Geometry: final body of the model. Coordinates: model frame, mm. A direction names the side the tool comes from. Give positions to 0.01 mm unless a question says otherwise; leave off trailing zeros. Write each loop counter-clockwise with the first axis right and the second up, starting at its lowest first coordinate (ties: lowest second). Pieces come first, ordered by that corner, then holes.
Q1. Reachability of faces 4 (the flat face through (15, -51, 0)), 5 (the flat face through (-1, 6, 4)), 6 (the flat face through (11, -54, 8)) from +Z, -Z, +X, -X, +Y, -Y: full face, straight path, thin tool, end or side. Return the list, or none.
Q2. Section C-C (y = -15.5). Return the cut outline in (x, z), plus the area to 3 significant figures.
Q3. Pin query (flat end, axial travel): pin 1 Ø2 at (x, z) = (8, 10.5) entering from +Y; pin 2 Ø3 at (y, z) = (1, 7) entering from -X; pin 3 Ø2 at (y, z) = (-28.5, -13) entering from -X. Return the tip coordinate at first contact, or that it passes through.
Q4. Section A-A (z = 0). Return the cut outline in (x, y), plus the area to 3 significant figures.
Q5. Section B-B (x = 0). Return the cut outline in (y, z), plus the area to 3 significant figures.
Q6. Line query: line 1 (Y direction, x = -12, z = 2.5); line 2 (Y direction, x = -13.5, z = -11.5); line 3 (Z direction, x = 13.5, y = -55). Output: solid intervals per line, ascending.
Q7. Section D-D (x = -7). Return the cut outline in (y, z), plus the area to 3 significant figures.
Q8. Mould query, pull axis X, two halves, no side actions, for faces 1 (the cylindrical face through (1.352, -55.19, 4.292)), 2 (the flat face through (11, -56.5, 0)), 3 (the cylindrical face through (-16.108, -38.325, -3.577)). Classes: +X half, -X half, draft (parallel to the pull), parting line (faces both ways), or undercut.
from build123d import *

# Parameters (mm, degrees)
SKETCH1_R           = 18.5
SKETCH1_R_2         = 16.5
SKETCH1_R_3         = 6
SKETCH1_R_4         = 4.5
SKETCH1_W           = 6
SKETCH1_H           = 16
SKETCH1_R_5         = 3
BOSS_EXTRUDE1_DEPTH = 26
BOSS_EXTRUDE2_START = -26
SKETCH1_3_R         = 16.5
BOSS_EXTRUDE2_DEPTH = 25
BOSS_EXTRUDE3_START = -56.5
SKETCH1_4_W         = 6
SKETCH1_4_H         = 16
BOSS_EXTRUDE3_DEPTH = 5.5
BOSS_EXTRUDE4_START = -51
SKETCH1_5_R         = 4.5
BOSS_EXTRUDE4_DEPTH = 8.5
SKETCH1_6_R         = 6
BOSS_EXTRUDE5_DEPTH = 6
BOSS_EXTRUDE6_START = 6
SKETCH1_7_R         = 3
BOSS_EXTRUDE6_DEPTH = 15


with BuildPart() as part:
    # Sketch1 → Boss-Extrude1 (new body)
    # profile 1 of 14: a face of its own
    with BuildSketch(Plane(origin=(0, 0, 0), x_dir=(1, 0, 0), z_dir=(0, 1, 0))):
        with Locations(Location((0, 0, 0), (0, 0, 270))):
            Circle(SKETCH1_R)
        Circle(SKETCH1_R_2, mode=Mode.SUBTRACT)
    # profile 2 of 14: a face of its own
    with BuildSketch(Plane(origin=(0, 0, 0), x_dir=(1, 0, 0), z_dir=(0, 1, 0))):
        with BuildLine():
            Line((14.43086969, -8), (8.43086969, -8))
            Line((8.43086969, -8), (8.43086969, 8))
            Line((8.43086969, 8), (14.43086969, 8))
            ThreePointArc((14.43086969, 8), (-16.5, 0), (14.43086969, -8))
        make_face()
        with BuildLine():
            ThreePointArc((3.822221213, -2.375), (5.428320517, -4.443960806), (6, -7))
            ThreePointArc((6, -7), (-2.556039194, -12.428320517), (-3.822221213, -2.375))
            ThreePointArc((-3.822221213, -2.375), (-1.234909823, 4.327239042), (4.5, 0))
            ThreePointArc((4.5, 0), (4.327239042, -1.234909823), (3.822221213, -2.375))
        make_face(mode=Mode.SUBTRACT)
    # profile 3 of 14: a face of its own
    with BuildSketch(Plane(origin=(0, 0, 0), x_dir=(1, 0, 0), z_dir=(0, 1, 0))):
        with Locations((0, -7)):
            Circle(SKETCH1_R_3)
    # profile 4 of 14: a face of its own
    with BuildSketch(Plane(origin=(0, 0, 0), x_dir=(1, 0, 0), z_dir=(0, 1, 0))):
        Circle(SKETCH1_R_4)
    # profile 5 of 14: a face of its own
    with BuildSketch(Plane(origin=(0, 0, 0), x_dir=(1, 0, 0), z_dir=(0, 1, 0))):
        with Locations((11.43086969, 0)):
            Rectangle(SKETCH1_W, SKETCH1_H)
    # profile 6 of 14: a face of its own
    with BuildSketch(Plane(origin=(0, 0, 0), x_dir=(1, 0, 0), z_dir=(0, 1, 0))):
        with BuildLine():
            Line((14.43086969, 8), (14.43086969, -8))
            ThreePointArc((14.43086969, -8), (15.974344273, -4.13162499), (16.5, 0))
            ThreePointArc((16.5, 0), (15.974344273, 4.13162499), (14.43086969, 8))
        make_face()
    # profile 7 of 14: a face of its own
    with BuildSketch(Plane(origin=(0, 0, 0), x_dir=(1, 0, 0), z_dir=(0, 1, 0))):
        Circle(SKETCH1_R_4)
    # profile 8 of 14: a face of its own
    with BuildSketch(Plane(origin=(0, 0, 0), x_dir=(1, 0, 0), z_dir=(0, 1, 0))):
        with Locations((0, -7)):
            Circle(SKETCH1_R_3)
        with Locations((0, -7)):
            Circle(SKETCH1_R_5, mode=Mode.SUBTRACT)
    # profile 9 of 14: a face of its own
    with BuildSketch(Plane(origin=(0, 0, 0), x_dir=(1, 0, 0), z_dir=(0, 1, 0))):
        Circle(SKETCH1_R_4)
    # profile 10 of 14: a face of its own
    with BuildSketch(Plane(origin=(0, 0, 0), x_dir=(1, 0, 0), z_dir=(0, 1, 0))):
        Circle(SKETCH1_R_4)
    # profile 11 of 14: a face of its own
    with BuildSketch(Plane(origin=(0, 0, 0), x_dir=(1, 0, 0), z_dir=(0, 1, 0))):
        with Locations((0, -7)):
            Circle(SKETCH1_R_3)
        with Locations((0, -7)):
            Circle(SKETCH1_R_5, mode=Mode.SUBTRACT)
    # profile 12 of 14: a face of its own
    with BuildSketch(Plane(origin=(0, 0, 0), x_dir=(1, 0, 0), z_dir=(0, 1, 0))):
        with Locations((0, -7)):
            Circle(SKETCH1_R_5)
    # profile 13 of 14: a face of its own
    with BuildSketch(Plane(origin=(0, 0, 0), x_dir=(1, 0, 0), z_dir=(0, 1, 0))):
        with Locations((0, -7)):
            Circle(SKETCH1_R_5)
    # profile 14 of 14: a face of its own
    with BuildSketch(Plane(origin=(0, 0, 0), x_dir=(1, 0, 0), z_dir=(0, 1, 0))):
        Circle(SKETCH1_R_4)
    extrude(amount=-BOSS_EXTRUDE1_DEPTH)

    # Sketch1<3> → Boss-Extrude2 (add)
    with BuildSketch(Plane(origin=(0, 0, 0), x_dir=(1, 0, 0), z_dir=(0, 1, 0)).offset(BOSS_EXTRUDE2_START)):
        with Locations(Location((0, 0, 0), (0, 0, 270))):
            Circle(SKETCH1_3_R)
    extrude(amount=-BOSS_EXTRUDE2_DEPTH)

    # Sketch1<4> → Boss-Extrude3 (add)
    with BuildSketch(Plane(origin=(0, 0, 0), x_dir=(1, 0, 0), z_dir=(0, 1, 0)).offset(BOSS_EXTRUDE3_START)):
        with Locations((11.43086969, 0)):
            Rectangle(SKETCH1_4_W, SKETCH1_4_H)
    extrude(amount=BOSS_EXTRUDE3_DEPTH)

    # Sketch1<5> → Boss-Extrude4 (add)
    with BuildSketch(Plane(origin=(0, 0, 0), x_dir=(1, 0, 0), z_dir=(0, 1, 0)).offset(BOSS_EXTRUDE4_START)):
        with Locations(Location((0, 0, 0), (0, 0, 270))):
            Circle(SKETCH1_5_R)
    extrude(amount=-BOSS_EXTRUDE4_DEPTH)

    # Sketch1<6> → Boss-Extrude5 (add)
    with BuildSketch(Plane(origin=(0, 0, 0), x_dir=(1, 0, 0), z_dir=(0, 1, 0))):
        with Locations(Location((0, -7, 0), (0, 0, 270))):
            Circle(SKETCH1_6_R)
    extrude(amount=BOSS_EXTRUDE5_DEPTH)

    # Sketch1<7> → Boss-Extrude6 (add)
    with BuildSketch(Plane(origin=(0, 0, 0), x_dir=(1, 0, 0), z_dir=(0, 1, 0)).offset(BOSS_EXTRUDE6_START)):
        with Locations(Location((0, -7, 0), (0, 0, 270))):
            Circle(SKETCH1_7_R)
    extrude(amount=BOSS_EXTRUDE6_DEPTH)


solid = part.part
Computed:
1. face 4: +Z, -Z, +X, -Y
1. face 5: +Y
1. face 6: +Z, +X, -X, -Y
2. outline: circle Ø37 at (0, 0)
2. area: 1,080 mm2
3. pin 1: stops at y = 0
3. pin 2: stops at x = -17.54
3. pin 3: stops at x = -11.32
4. outline: (-18.5, -26) - (-16.5, -26) - (-16.5, -51) - (-4.5, -51) - (-4.5, -59.5) - (4.5, -59.5) - (4.5, -51) - (8.43, -51) - (8.43, -56.5) - (14.43, -56.5) - (14.43, -51) - (16.5, -51) - (16.5, -26) - (18.5, -26) - (18.5, 0) - (-18.5, 0) - close
4. area: 1,900 mm2
5. outline: (-59.5, -4.5) - (-51, -4.5) - (-51, -16.5) - (-26, -16.5) - (-26, -18.5) - (0, -18.5) - (0, 1) - (6, 1) - (6, 4) - (21, 4) - (21, 10) - (6, 10) - (6, 13) - (0, 13) - (0, 18.5) - (-26, 18.5) - (-26, 16.5) - (-51, 16.5) - (-51, 4.5) - (-59.5, 4.5) - close
5. area: 2,030 mm2
6. line 1: y = -51 to 0
6. line 2: y = -26 to 0
6. line 3: z = -8 to 8
7. outline: (-51, -14.94) - (-26, -14.94) - (-26, -17.12) - (0, -17.12) - (0, 17.12) - (-26, 17.12) - (-26, 14.94) - (-51, 14.94) - close
7. area: 1,640 mm2
8. face 1: undercut
8. face 2: draft
8. face 3: parting line
